from build123d import *

# Parameters (mm, degrees)
SKETCH_1_W               = 25.57090008
SKETCH_1_H               = 8
SKETCH_1_R               = 1.5
EXTRUDE_1_DEPTH          = 60
SKETCH_2_W               = 25.57090008
SKETCH_2_H               = 8
EXTRUDE_2_DEPTH          = 60
SKETCH_3_W               = 28
SKETCH_3_H               = 44
CUT_EXTRUDE_1_DEPTH      = 69.0968921
FILLET_3_R               = 2
CUT_EXTRUDE_3_DEPTH      = 69.043275984
CUT_EXTRUDE_3_DEPTH_BACK = 69.043275984
SKETCH_5_W               = 19.965389019
SKETCH_5_H               = 10
SKETCH_5_W_2             = 8.378102734
SKETCH_5_W_3             = 2.578087264
SKETCH_5_W_4             = 4.306688818
FILLET_4_R               = 2
CUT_EXTRUDE_4_DEPTH      = 69.043275984
CUT_EXTRUDE_4_DEPTH_BACK = 69.043275984
SKETCH_6_W               = 44.193811727
SKETCH_6_H               = 36.690121775


with BuildPart() as part:
    # 草图1 → 凸台-拉伸1 (new body)
    with BuildSketch(Plane.XY):
        Rectangle(SKETCH_1_W, SKETCH_1_H)
        with Locations((-8, 0)):
            Circle(SKETCH_1_R, mode=Mode.SUBTRACT)
        with Locations(Location((8, 0, 0), (0, 0, 180))):
            Circle(SKETCH_1_R, mode=Mode.SUBTRACT)
    extrude(amount=EXTRUDE_1_DEPTH)

    # 草图2 → 凸台-拉伸2 (add)
    with BuildSketch(Plane(origin=(0, 0, 0), x_dir=(-1, 0, 0), z_dir=(0, 0, -1))):
        with BuildLine():
            Line((16.137009301, 11.124937293), (-26.558542517, 4.58378843))
            Line((-26.558542517, 4.58378843), (-17.833909304, -4.268253789))
            ThreePointArc((-17.833909304, -4.268253789), (-16.826188208, -4.941851182), (-15.634172765, -5.161702124))
            Line((-15.634172765, -5.161702124), (16.6770718, -4.481988152))
            Line((16.6770718, -4.481988152), (25.054954432, -4.542717367))
            ThreePointArc((25.054954432, -4.542717367), (27.868152877, -2.64179187), (27.105933567, 0.666776546))
            ThreePointArc((27.105933567, 0.666776546), (26.418024583, 1.322314845), (25.754738639, 2.002756605))
            Line((25.754738639, 2.002756605), (16.137009301, 11.124937293))
        make_face()
        Rectangle(SKETCH_2_W, SKETCH_2_H, mode=Mode.SUBTRACT)
    extrude(amount=-EXTRUDE_2_DEPTH)

    # 草图3 → 切除-拉伸1 (cut, through all)
    with BuildSketch(Plane(origin=(-0.101620306, -4.830676855, 0), x_dir=(0.9997788072376046, -0.02103179969837793, 0), z_dir=(-0.02103179969837793, -0.9997788072376046, 0))):
        with Locations((0, 30)):
            Rectangle(SKETCH_3_W, SKETCH_3_H)
    extrude(amount=-CUT_EXTRUDE_1_DEPTH, mode=Mode.SUBTRACT)

    # 圆角3
    fillet_3_edges = [part.edges().sort_by_distance(p)[0] for p in [
        (26.558542517, 4.58378843, 30),
    ]]
    fillet(fillet_3_edges, radius=FILLET_3_R)

    # 草图5 → 切除-拉伸3 (cut, two sides: drawn at the far end of the back side and taken through both)
    with BuildSketch(Plane(origin=(0.031610884, -4.360871013, 0), x_dir=(0.9999737288141071, 0.007248564106812576, 0), z_dir=(0.007248564106812577, -0.9999737288141072, 0)).offset(-CUT_EXTRUDE_3_DEPTH_BACK)):
        with Locations((-35.069918896, 47)):
            Rectangle(SKETCH_5_W, SKETCH_5_H)
        with Locations((-20.898173019, 47)):
            Rectangle(SKETCH_5_W_2, SKETCH_5_H)
        with Locations((-15.42007802, 47)):
            Rectangle(SKETCH_5_W_3, SKETCH_5_H)
        with Locations((-11.977689979, 47)):
            Rectangle(SKETCH_5_W_4, SKETCH_5_H)
    extrude(amount=CUT_EXTRUDE_3_DEPTH + CUT_EXTRUDE_3_DEPTH_BACK, mode=Mode.SUBTRACT)

    # 圆角4
    fillet_4_edges = [part.edges().sort_by_distance(p)[0] for p in [
        (14.017415967, 0.680655778, 52),
        (14.017415967, 0.680655778, 8),
        (-13.937599421, 3.113545967, 8),
    ]]
    fillet(fillet_4_edges, radius=FILLET_4_R)

    # 草图6 → 切除-拉伸4 (cut, two sides: drawn at the far end of the back side and taken through both)
    with BuildSketch(Plane(origin=(0.031610884, -4.360871013, 0), x_dir=(0.9999737288141071, 0.007248564106812576, 0), z_dir=(0.007248564106812577, -0.9999737288141072, 0)).offset(-CUT_EXTRUDE_4_DEPTH_BACK)):
        with Locations((-28.444987659, 26.345060888)):
            Rectangle(SKETCH_6_W, SKETCH_6_H)
    extrude(amount=CUT_EXTRUDE_4_DEPTH + CUT_EXTRUDE_4_DEPTH_BACK, mode=Mode.SUBTRACT)


solid = part.part
Design review of the part built by this model. Coordinates are the model's own, in mm. A direction names the side the tool comes from. Round coordinates to 2 decimals unless told otherwise and drop trailing zeros. Loops run counter-clockwise (first coordinate to the right, second up) from the corner with the lowest first, then second, coordinate; pieces in that order, holes last. Notation, with made-up numbers: (30, 56.5) - (38, 56.5) arc R13 ccw to (38, 69.5) - close; hole circle Ø2 at (82, 34). An arc over 180 degrees is marked (long way). One line per question, with ' | ' between items.
1. Clearance check with flat-ended pins moving along their axes: P1, Ø2, axis at y = -2, z = 25.5, coming from the -X side; P2, Ø4, axis at x = -8, y = 0, coming from the -Z side. State where each tip first meets the part, or that it passes through.
Results are:
P1: stops at x = 13.94 | P2: stops at z = 0
2. We need section D-D, the plane y = 0. State how many separate pieces and enclosed holes the cut face has, and give its area (3 significant figures).
Results are:
separate pieces: 5 | enclosed holes: 0 | area: 1,050 mm²
3. For L1, parallel to Z at x = -7.5, y = 8.25; L2, parallel to Y at x = -8, z = 5.5; L3, parallel to X at y = 0.5, z = 54, list the stretches that pass through material, from the lowest coordinate up. Write a range as [from, to].
Results are:
L1: z = [0, 8], [52, 60] | L2: y = [-4.66, -1.5], [1.5, 9.88] | L3: x = [-27.27, -9.41], [-6.59, 6.59], [9.41, 22.53]
4. We need section C-C, the plane x = -8. State the section outline as (y, z) points.
Results are:
outline: (-4.66, 0) - (-1.5, 0) - (-1.5, 8) - (-4.66, 8) - close; (-4.66, 52) - (-1.5, 52) - (-1.5, 60) - (-4.66, 60) - close; (1.5, 0) - (9.88, 0) - (9.88, 8) - (1.5, 8) - close; (1.5, 52) - (9.88, 52) - (9.88, 60) - (1.5, 60) - close
5. We need section B-B, the plane x = 10.5. State the section outline as (y, z) points.
Results are:
outline: (-5.05, 0) - (7.04, 0) - (7.04, 8) - (-5.05, 8) - close; (-5.05, 52) - (7.04, 52) - (7.04, 60) - (-5.05, 60) - close
6. Draft analysis for pull direction X (two halves, no side actions). For faces 1 (the face through (9.5, -0.07, 3.94)), 2 (the face through (20.864, -1.194, 29.58)), 3 (the face through (9.5, -0.07, 55.94)), 4 (the face through (13.45, 0.91, 8.6)), state which applies: released by +X, released by -X, zero draft, split by the parting line, or undercut.
Results are:
face 1: undercut | face 2: released by +X | face 3: undercut | face 4: released by -X
7. We need section A-A, the plane z = 53. State the section outline as (x, y) points.
Results are:
outline: (-27.11, 0.67) arc R3 ccw to (-25.05, -4.54) - (-16.68, -4.48) - (15.63, -5.16) arc R3 ccw to (17.83, -4.27) - (23.81, 1.8) arc R2 ccw to (22.69, 5.18) - (-16.14, 11.12) - (-25.75, 2) arc R25.78 cw to start; hole circle Ø3 at (-8, 0); hole circle Ø3 at (8, 0)
8. For faces 5 (the face through (-26.43, 1.31, 3.94)), 6 (the face through (13.42, 0.91, 51.43)), 7 (the face through (-8, 3, 52)), list the 3-axis set-ups (+Z, -Z, +X, -X, +Y, -Y) from which the entire face can be reached by the end or side of a thin tool; tool diameter is ignored.
Results are:
face 5: +Z, -Z, -X, +Y | face 6: -X, +Y | face 7: -X, +Y, -Y
